Autodesk Inventor part; units mm, degrees
ref_plane "Work Plane1" through (9.5307, 0, 0) normal (0, 0, 1) x (-1, 0, 0)
ref_plane "YZ Plane" through (0, 0, 0) normal (1, 0, 0) x (0, 1, 0)
ref_plane "XZ Plane" through (0, 0, 0) normal (0, 1, 0) x (-1, 0, 0)
sketch "Sketch1" plane through (0, 0, 0) normal (1, 0, 0) x (0, 1, 0)
  line L0 (1.5877, -2.75) -> (-1.5877, -2.75)
  line L1 (-1.5877, -2.75) -> (-3.1754, 0)
  line L2 (-3.1754, 0) -> (-1.5877, 2.75)
  line L3 (-1.5877, 2.75) -> (1.5877, 2.75)
  line L4 (1.5877, 2.75) -> (3.1754, 0)
  line L5 (3.1754, 0) -> (1.5877, -2.75)
  point P0 (0, 0)
  point P1 (0, 0)
  dimension "d0" = 6.3509
extrude "Body" add sketch "Sketch1" along normal blind 2.15
sketch "Sketch2" plane through (2.15, 0, 0) normal (1, 0, 0) x (0, 0, -1)
  circle A0 centre (0, 0) radius 2.285
  dimension "d7" = 4.57
extrude "Ring" add sketch "Sketch2" along normal blind 2.35
sketch "Sketch3" plane through (0, 0, 0) normal (0, 0, 1) x (1, 0, 0)
  line L0 (0, 1.5877) -> (0, 3.1754)
  line L1 (0, 3.1754) -> (2.15, 3.1754)
  line L2 (2.15, 1.5877) -> (2.15, 3.1754)
  line L3 (-0.43, 0) -> (2.58, 0)
  line L4 (0, 2.285) -> (0.5141, 3.1754)
  line L5 (1.6359, 3.1754) -> (2.15, 2.285)
  dimension "d3" = 30
  dimension "d4" = 30
  dimension "d5" = 4.57
  dimension "d6" = 4.57
revolve "Chamfer1" cut sketch "Sketch3" angle 360 about axis through (-10, 0, 0) along (1, 0, 0)
sketch "Sketch4" plane through (0, 0, 0) normal (-1, 0, 0) x (0, 0, 1)
  line L0 (0, -4.4456) -> (0, 4.4456)
  line L1 (-3.85, 0) -> (3.85, 0)
  point P0 (0, 0)
hole "Thread" at (0, 0, 0) direction (1, 0, 0) diameter 2.459 end through all
chamfer "Chamfer2" distance 0.2706 angle 30 1 edges at (0, 0, -1.2295) measured on face at (0, 1.908, -0.2317)
chamfer "Chamfer3" distance 0.2706 angle 30 1 edges at (4.5, 0, -1.2295) measured on face at (4.5, -0.2804, -1.8991)
ref_plane "Work Plane1" through (9.5307, 0, 0) normal (0, 0, 1) x (-1, 0, 0)
fillet "Fillet1" radius 0.7 1 edges at (4.5, 0, 2.285)
equation "\"d0\" = 1.1547 * SW"
equation "\"d1\" = KOH1"
equation "\"d7\" = SD2"
equation "\"d8\" = KOH - KOH1"
equation "\"d3\" = ANG1"
equation "\"d4\" = ANG2"
equation "\"d5\" = SW0"
equation "\"d6\" = SW01"
equation "\"d10\" = -0.5 * GD1 + 0.5 * NND"
equation "\"d46\" = -0.5 * GD1 + 0.5 * NND"
equation "\"d12\" = -0.5 * GD1 + 0.5 * NND"
equation "\"d47\" = -0.5 * GD1 + 0.5 * NND"
equation "\"ANG1\" = 30deg"
equation "\"ANG2\" = 30deg"
equation "\"NND\" = 3"
equation "\"KOH1\" = 2.15"
equation "\"KOH\" = 4.5"
equation "\"SW\" = 5.5"
equation "\"SW0\" = 4.57"
equation "\"SW01\" = SW0"
equation "\"SD2\" = SW0"
equation "\"GUL\" = 0.541266 * PTC"
equation "\"THREADDIA\" = 3"
equation "\"TOA\" = 30deg"
equation "\"PTC\" = 0.5"
equation "\"E0\" = 1.155 * SW"
equation "\"GAL\" = 0.541266 * PTC"
properties part number "ISO 7040 - M3" material "Steel"
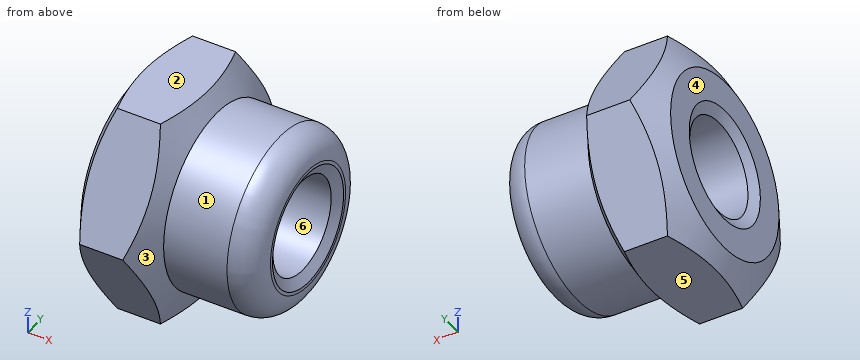
For this review, take the finished solid that the model builds, in its own axes (mm). Face numbers are marked on the shaded views. A direction names the side the tool comes from. Coordinates: 2 decimals unless noted, no trailing zeros. Loops run counter-clockwise (first coordinate to the right, second up) from the corner with the lowest first, then second, coordinate; pieces in that order, holes last.
1. Add section B-B, the plane x = 1.75. Give the boundary of the cut face in (y, z).
2. For the marked faces 1 and 2, list the 3-axis set-ups (+Z, -Z, +X, -X, +Y, -Y) from which the entire face can be reached by the end or side of a thin tool; tool diameter is ignored.
3. Insertion check: P1, Ø1, axis at x = 1, z = -1, coming from the +Y side; P2, Ø1.5, axis at y = -1, z = -0.5, coming from the +X side; P3, Ø2, axis at y = 0, z = 0, coming from the +X side. Each pin has a flat end and moves straight along its axis. Give the tip position at first contact, or say it passes through.
4. Add section C-C, the plane x = 3.7. Give the boundary of the cut face in (y, z) (1 decimal).
5. Mouldability with a two-part tool opening along Z and no side actions: class the marked faces 3, 4, 5 and 6 as +Z half, -Z half, draft (parallel to the pull), parting line (faces both ways), or undercut.
6. For line 1 (Z direction, x = 1.85, y = 0); line 2 (Y direction, x = 3.15, z = 0) (1 decimal), list the stretches that pass through material, from the lowest coordinate up.
Result:
1. outline: (-2.95, -0.39) - (-1.81, -2.36) arc R2.98 ccw to (-1.14, -2.75) - (1.14, -2.75) arc R2.98 ccw to (1.81, -2.36) - (2.95, -0.39) arc R2.98 ccw to (2.95, 0.39) - (1.81, 2.36) arc R2.98 ccw to (1.14, 2.75) - (-1.14, 2.75) arc R2.98 ccw to (-1.81, 2.36) - (-2.95, 0.39) arc R2.98 ccw to start; hole circle Ø2.46 at (0, 0)
2. face 1: +X
2. face 2: +Z, +X, -X, +Y, -Y
3. P1: stops at y = 2.89
3. P2: stops at x = 4.5
3. P3: passes through
4. outline: circle Ø4.6 at (0, 0); hole circle Ø2.5 at (0, 0)
5. face 3: parting line
5. face 4: draft
5. face 5: -Z half
5. face 6: undercut
6. line 1: z = -2.75 to -1.23, 1.23 to 2.75
6. line 2: y = -2.3 to -1.2, 1.2 to 2.3
